Geometry: final body of the model. Coordinates: model frame, mm. Round coordinates to 2 decimals unless told otherwise and drop trailing zeros. Loops run counter-clockwise (first coordinate to the right, second up) from the corner with the lowest first, then second, coordinate; pieces in that order, holes last. Notation, with made-up numbers: (18, -38) - (65, -38) arc R22 ccw to (65, -8) - close; hole circle Ø5 at (15, -34.75). An arc over 180 degrees is marked (long way). Answer as CSV lines item,"result".
from build123d import *

# Parameters (mm, degrees)
SKETCH1_W           = 482.6
SKETCH1_H           = 254
BOSS_EXTRUDE1_DEPTH = 3.175
FILLET1_R           = 6.35
CUT_EXTRUDE1_REACH  = 274.754
SKETCH3_R           = 3.05
CUT_EXTRUDE2_DEPTH  = 273.754491255


with BuildPart() as part:
    # Sketch1 → Boss-Extrude1 (new, symmetric)
    with BuildSketch(Plane(origin=(0, 0, 0), x_dir=(1, 0, 0), z_dir=(0, 1, 0))):
        Rectangle(SKETCH1_W, SKETCH1_H)
    extrude(amount=BOSS_EXTRUDE1_DEPTH, both=True)

    # Fillet1
    fillet1_edges = [part.edges().sort_by_distance(p)[0] for p in [
        (241.3, 0, 127),
        (-241.3, 0, 127),
        (-241.3, 0, -127),
        (241.3, 0, -127),
    ]]
    fillet(fillet1_edges, radius=FILLET1_R)

    # Sketch2 → Cut-Extrude1 (cut, up to next)
    with BuildSketch(Plane(origin=(0, 3.175, 0), x_dir=(1, 0, 0), z_dir=(0, 1, 0)), mode=Mode.PRIVATE) as cut_extrude1_sk1:
        with BuildLine():
            Line((227.25, -82.55), (227.25, -107.95))
            ThreePointArc((227.25, -107.95), (222.25, -112.95), (217.25, -107.95))
            Line((217.25, -107.95), (217.25, -82.55))
            ThreePointArc((217.25, -82.55), (222.25, -77.55), (227.25, -82.55))
        make_face()
    cut_extrude1_tool1 = extrude(cut_extrude1_sk1.sketch, amount=-CUT_EXTRUDE1_REACH, mode=Mode.PRIVATE) & part.part
    # Sketch2 → Cut-Extrude1 (cut, up to next)
    with BuildSketch(Plane(origin=(0, 3.175, 0), x_dir=(1, 0, 0), z_dir=(0, 1, 0)), mode=Mode.PRIVATE) as cut_extrude1_sk2:
        with BuildLine():
            Line((227.25, -44.45), (227.25, -19.05))
            ThreePointArc((227.25, -19.05), (222.25, -14.05), (217.25, -19.05))
            Line((217.25, -19.05), (217.25, -44.45))
            ThreePointArc((217.25, -44.45), (222.25, -49.45), (227.25, -44.45))
        make_face()
    cut_extrude1_tool2 = extrude(cut_extrude1_sk2.sketch, amount=-CUT_EXTRUDE1_REACH, mode=Mode.PRIVATE) & part.part
    # Sketch2 → Cut-Extrude1 (cut, up to next)
    with BuildSketch(Plane(origin=(0, 3.175, 0), x_dir=(1, 0, 0), z_dir=(0, 1, 0)), mode=Mode.PRIVATE) as cut_extrude1_sk3:
        with BuildLine():
            Line((227.25, 44.45), (227.25, 19.05))
            ThreePointArc((227.25, 19.05), (222.25, 14.05), (217.25, 19.05))
            Line((217.25, 19.05), (217.25, 44.45))
            ThreePointArc((217.25, 44.45), (222.25, 49.45), (227.25, 44.45))
        make_face()
    cut_extrude1_tool3 = extrude(cut_extrude1_sk3.sketch, amount=-CUT_EXTRUDE1_REACH, mode=Mode.PRIVATE) & part.part
    # Sketch2 → Cut-Extrude1 (cut, up to next)
    with BuildSketch(Plane(origin=(0, 3.175, 0), x_dir=(1, 0, 0), z_dir=(0, 1, 0)), mode=Mode.PRIVATE) as cut_extrude1_sk4:
        with BuildLine():
            Line((227.25, 82.55), (227.25, 107.95))
            ThreePointArc((227.25, 107.95), (222.25, 112.95), (217.25, 107.95))
            Line((217.25, 107.95), (217.25, 82.55))
            ThreePointArc((217.25, 82.55), (222.25, 77.55), (227.25, 82.55))
        make_face()
    cut_extrude1_tool4 = extrude(cut_extrude1_sk4.sketch, amount=-CUT_EXTRUDE1_REACH, mode=Mode.PRIVATE) & part.part
    # Sketch2 → Cut-Extrude1 (cut, up to next)
    with BuildSketch(Plane(origin=(0, 3.175, 0), x_dir=(1, 0, 0), z_dir=(0, 1, 0)), mode=Mode.PRIVATE) as cut_extrude1_sk5:
        with BuildLine():
            Line((-227.25, 82.55), (-227.25, 107.95))
            ThreePointArc((-227.25, 107.95), (-222.25, 112.95), (-217.25, 107.95))
            Line((-217.25, 107.95), (-217.25, 82.55))
            ThreePointArc((-217.25, 82.55), (-222.25, 77.55), (-227.25, 82.55))
        make_face()
    cut_extrude1_tool5 = extrude(cut_extrude1_sk5.sketch, amount=-CUT_EXTRUDE1_REACH, mode=Mode.PRIVATE) & part.part
    # Sketch2 → Cut-Extrude1 (cut, up to next)
    with BuildSketch(Plane(origin=(0, 3.175, 0), x_dir=(1, 0, 0), z_dir=(0, 1, 0)), mode=Mode.PRIVATE) as cut_extrude1_sk6:
        with BuildLine():
            Line((-227.25, 44.45), (-227.25, 19.05))
            ThreePointArc((-227.25, 19.05), (-222.25, 14.05), (-217.25, 19.05))
            Line((-217.25, 19.05), (-217.25, 44.45))
            ThreePointArc((-217.25, 44.45), (-222.25, 49.45), (-227.25, 44.45))
        make_face()
    cut_extrude1_tool6 = extrude(cut_extrude1_sk6.sketch, amount=-CUT_EXTRUDE1_REACH, mode=Mode.PRIVATE) & part.part
    # Sketch2 → Cut-Extrude1 (cut, up to next)
    with BuildSketch(Plane(origin=(0, 3.175, 0), x_dir=(1, 0, 0), z_dir=(0, 1, 0)), mode=Mode.PRIVATE) as cut_extrude1_sk7:
        with BuildLine():
            Line((-227.25, -44.45), (-227.25, -19.05))
            ThreePointArc((-227.25, -19.05), (-222.25, -14.05), (-217.25, -19.05))
            Line((-217.25, -19.05), (-217.25, -44.45))
            ThreePointArc((-217.25, -44.45), (-222.25, -49.45), (-227.25, -44.45))
        make_face()
    cut_extrude1_tool7 = extrude(cut_extrude1_sk7.sketch, amount=-CUT_EXTRUDE1_REACH, mode=Mode.PRIVATE) & part.part
    # Sketch2 → Cut-Extrude1 (cut, up to next)
    with BuildSketch(Plane(origin=(0, 3.175, 0), x_dir=(1, 0, 0), z_dir=(0, 1, 0)), mode=Mode.PRIVATE) as cut_extrude1_sk8:
        with BuildLine():
            Line((-227.25, -82.55), (-227.25, -107.95))
            ThreePointArc((-227.25, -107.95), (-222.25, -112.95), (-217.25, -107.95))
            Line((-217.25, -107.95), (-217.25, -82.55))
            ThreePointArc((-217.25, -82.55), (-222.25, -77.55), (-227.25, -82.55))
        make_face()
    cut_extrude1_tool8 = extrude(cut_extrude1_sk8.sketch, amount=-CUT_EXTRUDE1_REACH, mode=Mode.PRIVATE) & part.part
    add(cut_extrude1_tool1.solids().sort_by_distance((222.25, 3.175, 95.25))[0], mode=Mode.SUBTRACT)
    add(cut_extrude1_tool2.solids().sort_by_distance((222.25, 3.175, 31.75))[0], mode=Mode.SUBTRACT)
    add(cut_extrude1_tool3.solids().sort_by_distance((222.25, 3.175, -31.75))[0], mode=Mode.SUBTRACT)
    add(cut_extrude1_tool4.solids().sort_by_distance((222.25, 3.175, -95.25))[0], mode=Mode.SUBTRACT)
    add(cut_extrude1_tool5.solids().sort_by_distance((-222.25, 3.175, -95.25))[0], mode=Mode.SUBTRACT)
    add(cut_extrude1_tool6.solids().sort_by_distance((-222.25, 3.175, -31.75))[0], mode=Mode.SUBTRACT)
    add(cut_extrude1_tool7.solids().sort_by_distance((-222.25, 3.175, 31.75))[0], mode=Mode.SUBTRACT)
    add(cut_extrude1_tool8.solids().sort_by_distance((-222.25, 3.175, 95.25))[0], mode=Mode.SUBTRACT)

    # Sketch3 → Cut-Extrude2 (cut, through all)
    with BuildSketch(Plane(origin=(0, 3.175, 0), x_dir=(1, 0, 0), z_dir=(0, 1, 0))):
        with Locations(Location((-50.8, 98.956, 0), (0, 0, 270))):
            Circle(SKETCH3_R)
        with Locations(Location((-50.8, 63.956, 0), (0, 0, 270))):
            Circle(SKETCH3_R)
        with Locations(Location((-50.8, 28.956, 0), (0, 0, 270))):
            Circle(SKETCH3_R)
    extrude(amount=-CUT_EXTRUDE2_DEPTH, mode=Mode.SUBTRACT)


solid = part.part
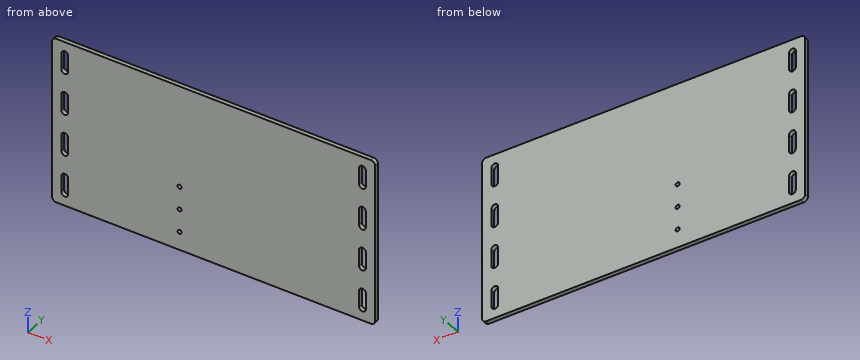
(1) Section A-A (z = 99). Output: boundary loops of the cut face in (x, y) (3 decimals).
Findings below:
outline,"(-241.3, -3.175) - (-227.25, -3.175) - (-227.25, 3.175) - (-241.3, 3.175) - close; (-217.25, -3.175) - (217.25, -3.175) - (217.25, 3.175) - (-217.25, 3.175) - close; (227.25, -3.175) - (241.3, -3.175) - (241.3, 3.175) - (227.25, 3.175) - close"
(2) Section B-B (y = -1.75). Give the number of separate pieces and of enclosed holes in the cut face, and give its area (3 significant figures).
Findings below:
separate pieces,"1"
enclosed holes,"11"
area,"120,000 mm2"
(3) Pin query (flat end, axial travel): P1, Ø3.5, axis at x = -50.8, z = -63.956, coming from the -Y side. Return the tip coordinate at first contact, or that it passes through.
Findings below:
P1,"through"
(4) Material intervals for line 1 along X through (y, z) = (2.25, 86), sorted ascending.
Findings below:
line 1,"-241.3 to -227.25, -217.25 to 217.25, 227.25 to 241.3"
